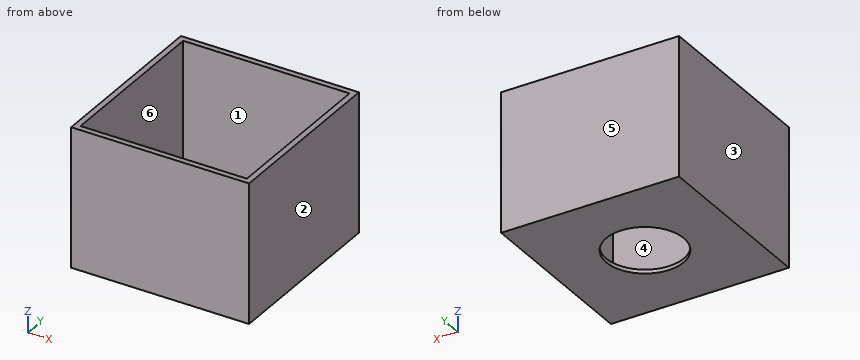
from build123d import *

# Parameters (mm, degrees)
ESQUISSE1_W             = 46
ESQUISSE1_H             = 46
BOSS_EXTRU_1_DEPTH      = 36
ESQUISSE2_W             = 43
ESQUISSE2_H             = 43
ENL_V_MAT_EXTRU_1_DEPTH = 35
ESQUISSE3_R             = 10
ENL_V_MAT_EXTRU_2_DEPTH = 35


with BuildPart() as part:
    # Esquisse1 → Boss.-Extru.1 (new body)
    with BuildSketch(Plane.XY):
        Rectangle(ESQUISSE1_W, ESQUISSE1_H)
    extrude(amount=BOSS_EXTRU_1_DEPTH)

    # Esquisse2 → Enlèv. mat.-Extru.1 (cut)
    with BuildSketch(Plane.XY.offset(36)):
        Rectangle(ESQUISSE2_W, ESQUISSE2_H)
    extrude(amount=-ENL_V_MAT_EXTRU_1_DEPTH, mode=Mode.SUBTRACT)

    # Esquisse3 → Enlèv. mat.-Extru.2 (cut)
    with BuildSketch(Plane(origin=(0, 0, 0), x_dir=(-1, 0, 0), z_dir=(0, 0, -1))):
        Circle(ESQUISSE3_R)
    extrude(amount=-ENL_V_MAT_EXTRU_2_DEPTH, mode=Mode.SUBTRACT)


solid = part.part
Geometry: final body of the model. Coordinates: model frame, mm. Face numbers are marked on the shaded views. A direction names the side the tool comes from. Round coordinates to 2 decimals unless told otherwise and drop trailing zeros. Loops run counter-clockwise (first coordinate to the right, second up) from the corner with the lowest first, then second, coordinate; pieces in that order, holes last.
Q1. Section A-A on y = 0. Return loops of the section in (x, z), plus the area to 3 significant figures.
Q2. Pull-direction query (X, two-part tool) for the marked faces 1, 2, 3 and 4; classes: released by +X, released by -X, zero draft, split by the parting line, or undercut.
Q3. Access query for the marked faces 5 and 6. Directions: +Z, -Z, +X, -X, +Y, -Y. A direction counts if a zero-diameter tool reaches every point of the face in a straight line with its end or side. Return the directions, or none.
Q4. Pin query (flat end, axial travel): P1, Ø21.5, axis at x = -4, y = -2, coming from the +Z side; P2, Ø18, axis at x = 0, y = 0, coming from the +Z side. Return the tip coordinate at first contact, or that it passes through.
Q5. Section C-C on z = 15.5. Return loops of the section in (x, y), plus the area to 3 significant figures.
Q6. Section D-D on y = 19.5. Return loops of the section in (x, z), plus the area to 3 significant figures.
Q7. Material intervals for L1, parallel to X at y = 10.5, z = 21.5; L2, parallel to Y at x = 0, z = 0.45, sorted ascending.
Evaluation:
1. outline: (-23, 0) - (-10, 0) - (-10, 1) - (-21.5, 1) - (-21.5, 36) - (-23, 36) - close; (10, 0) - (23, 0) - (23, 36) - (21.5, 36) - (21.5, 1) - (10, 1) - close
1. area: 131 mm2
2. face 1: undercut
2. face 2: released by +X
2. face 3: released by -X
2. face 4: undercut
3. face 5: +Z, -Z, +X, -X, +Y
3. face 6: +Z
4. P1: stops at z = 1
4. P2: passes through
5. outline: (-23, -23) - (23, -23) - (23, 23) - (-23, 23) - close; hole (-21.5, -21.5) - (21.5, -21.5) - (21.5, 21.5) - (-21.5, 21.5) - close
5. area: 267 mm2
6. outline: (-23, 0) - (23, 0) - (23, 36) - (21.5, 36) - (21.5, 1) - (-21.5, 1) - (-21.5, 36) - (-23, 36) - close
6. area: 151 mm2
7. L1: x = -23 to -21.5, 21.5 to 23
7. L2: y = -23 to -10, 10 to 23
